Verification items for the finished model (mm, model axes). A direction names the side the tool comes from. Give positions to 0.01 mm unless a question says otherwise; leave off trailing zeros. Loops run counter-clockwise (first coordinate to the right, second up) from the corner with the lowest first, then second, coordinate; pieces in that order, holes last. Notation, with made-up numbers: M 32,9 L 70,9 A24 cw 70,32 Z; hole C -14,54 d11. An arc over 180 degrees is marked long. Use a Markdown table: item, result.
from build123d import *

# Parameters (mm, degrees)
SKETCH_1_R          = 2.75
EXTRUDE_1_DEPTH     = 5
SKETCH_2_R          = 2.5
CUT_EXTRUDE_1_DEPTH = 4.7
SKETCH_3_R          = 1.5
CUT_EXTRUDE_2_DEPTH = 4.7
EXTRUDE_START       = -2
SKETCH_4_R          = 1.25
EXTRUDE_3_DEPTH     = 2
SKETCH_5_R          = 1.25
CUT_EXTRUDE_3_DEPTH = 10


with BuildPart() as part:
    # 草图1 → 凸台-拉伸1 (new body)
    with BuildSketch(Plane.XY):
        Circle(SKETCH_1_R)
    extrude(amount=EXTRUDE_1_DEPTH)

    # 草图2 → 切除-拉伸1 (cut)
    with BuildSketch(Plane(origin=(0, 0, 0), x_dir=(-1, 0, 0), z_dir=(0, 0, -1))):
        Circle(SKETCH_2_R)
    extrude(amount=-CUT_EXTRUDE_1_DEPTH, mode=Mode.SUBTRACT)

    # 草图3 → 切除-拉伸2 (cut)
    with BuildSketch(Plane.XY.offset(5)):
        Circle(SKETCH_3_R)
    extrude(amount=-CUT_EXTRUDE_2_DEPTH, mode=Mode.SUBTRACT)

    # 草图4 → 凸台-拉伸3 (add)
    with BuildSketch(Plane.XY.offset(5).offset(EXTRUDE_START)):
        with BuildLine():
            Line((29.765180985, 1.590978823), (0.10719348, 2.747910035))
            ThreePointArc((0.10719348, 2.747910035), (1.982079977, 1.906268335), (2.75, 0))
            ThreePointArc((2.75, 0), (1.982079977, -1.906268335), (0.10719348, -2.747910035))
            Line((0.10719348, -2.747910035), (29.765180985, -1.590978823))
            ThreePointArc((29.765180985, -1.590978823), (31.29530721, 0), (29.765180985, 1.590978823))
        make_face()
        with Locations((14.11, 0)):
            Circle(SKETCH_4_R, mode=Mode.SUBTRACT)
        with Locations((24.43, 0)):
            Circle(SKETCH_4_R, mode=Mode.SUBTRACT)
        with Locations((29.8799998, 0.003455751)):
            Circle(SKETCH_4_R, mode=Mode.SUBTRACT)
    extrude(amount=EXTRUDE_3_DEPTH)

    # 草图5 → 切除-拉伸3 (cut)
    with BuildSketch(Plane.XY.offset(5)):
        with Locations((19.56, 0)):
            Circle(SKETCH_5_R)
    extrude(amount=-CUT_EXTRUDE_3_DEPTH, mode=Mode.SUBTRACT)


solid = part.part
(1) Set-up check for faces 1 (the flat face through (14.729, -2.178, 3.986)), 2 (the flat face through (0, -2, 4.7)): record each of +Z, -Z, +X, -X, +Y, -Y from which the full face is reachable in a straight line by a thin tool's end or side.
Results below:
| item | result |
|---|---|
| face 1 | +Z, -Z, +X, -Y |
| face 2 | -Z |
(2) Cross-section at B-B on x = 19.56. Record the cut outline in (y, z).
Results below:
| item | result |
|---|---|
| outline | M -1.99,3 L -1.25,3 L -1.25,5 L -1.99,5 Z; M 1.25,3 L 1.99,3 L 1.99,5 L 1.25,5 Z |
(3) Draft check along X on faces 3 (the cylindrical face through (-2.747, 0.121, 1.909)), 4 (the cylindrical face through (-1.19, -0.91, 4.85)), 5 (the cylindrical face through (28.63, 0.06, 3.99)), 6 (the cylindrical face through (31.295, -0.034, 3.986)). Enter one of: +X half, -X half, draft (parallel to the pull), parting line (faces both ways), or undercut.
Results below:
| item | result |
|---|---|
| face 3 | parting line |
| face 4 | undercut |
| face 5 | undercut |
| face 6 | +X half |
(4) Cross-section at D-D on y = -2.2. Record the cut outline in (x, z), then the cut area to 3 significant figures.
Results below:
| item | result |
|---|---|
| outline | M -1.65,0 L -1.19,0 L -1.19,4.7 L 1.19,4.7 L 1.19,0 L 1.65,0 L 1.65,3 L 14.15,3 L 14.15,5 L -1.65,5 Z |
| area | 30.3 mm^2 |
(5) Cross-section at A-A on y = -0.8. State how many separate pieces and enclosed holes the cut face has, then the cut area to 3 significant figures.
Results below:
| item | result |
|---|---|
| separate pieces | 6 |
| enclosed holes | 0 |
| area | 44.8 mm^2 |
(6) Gauge pin test, flat end, axial feed: P1, Ø1.6, axis at x = 15.5, y = -1, coming from the -Z side. Record the tip position at first contact, or that the pin passes through.
Results below:
| item | result |
|---|---|
| P1 | z = 3 |
(7) Cross-section at C-C on z = 2.3. Record the cut outline in (x, y).
Results below:
| item | result |
|---|---|
| outline | C 0,0 d5.5; hole C 0,0 d5 |
(8) Material ranges on line 1 (Y direction, x = 0, z = 3.25); line 2 (Z direction, x = 29, y = 1.25); line 3 (X direction, y = -1, z = 2.75), recorded low to high.
Results below:
| item | result |
|---|---|
| line 1 | -2.75 to -2.5, 2.5 to 2.75 |
| line 2 | 3 to 5 |
| line 3 | -2.56 to -2.29, 2.29 to 2.56 |
